For this review, take the finished solid that the model builds, in its own axes (mm). A direction names the side the tool comes from. Give positions to 0.01 mm unless a question says otherwise; leave off trailing zeros. Loops run counter-clockwise (first coordinate to the right, second up) from the corner with the lowest first, then second, coordinate; pieces in that order, holes last. Notation, with made-up numbers: (58.5, 65.5) - (89.5, 65.5) arc R26 ccw to (89.5, 79.5) - close; hole circle Ø3 at (46, -13). An arc over 180 degrees is marked (long way). Put each result on its own line as item: value.
from build123d import *

# Parameters (mm, degrees)
ESQUISSE1_R        = 1.75
BOSS_EXTRU_1_DEPTH = 10
BOSS_EXTRU_2_START = 25
ESQUISSE2_R        = 4
BOSS_EXTRU_2_DEPTH = 10
CHANFREIN1_SIZE    = 2
CONG_1_R           = 2


with BuildPart() as part:
    # Esquisse1 → Boss.-Extru.1 (new body)
    with BuildSketch(Plane.XY):
        with BuildLine():
            Line((-2.952917385, 110.865117237), (48.5, 73.209447125))
            Line((48.5, 73.209447125), (48.5, 41.690552875))
            Line((48.5, 41.690552875), (-2.952917385, 4.034882763))
            ThreePointArc((-2.952917385, 4.034882763), (-4.034882763, -2.952917385), (2.952917385, -4.034882763))
            Line((2.952917385, -4.034882763), (56.966203668, 35.494585987))
            Line((56.966203668, 35.494585987), (100.033796332, 35.494585987))
            Line((100.033796332, 35.494585987), (154.047082615, -4.034882763))
            ThreePointArc((154.047082615, -4.034882763), (161.034882763, -2.952917385), (159.952917385, 4.034882763))
            Line((159.952917385, 4.034882763), (108.5, 41.690552875))
            Line((108.5, 41.690552875), (108.5, 73.209447125))
            Line((108.5, 73.209447125), (159.952917385, 110.865117237))
            ThreePointArc((159.952917385, 110.865117237), (161.034882763, 117.852917385), (154.047082615, 118.934882763))
            Line((154.047082615, 118.934882763), (100.033796332, 79.405414013))
            Line((100.033796332, 79.405414013), (56.966203668, 79.405414013))
            Line((56.966203668, 79.405414013), (2.952917385, 118.934882763))
            ThreePointArc((2.952917385, 118.934882763), (-4.034882763, 117.852917385), (-2.952917385, 110.865117237))
        make_face()
        Circle(ESQUISSE1_R, mode=Mode.SUBTRACT)
        with Locations((0, 114.9)):
            Circle(ESQUISSE1_R, mode=Mode.SUBTRACT)
        with Locations((157, 0)):
            Circle(ESQUISSE1_R, mode=Mode.SUBTRACT)
        with Locations((157, 114.9)):
            Circle(ESQUISSE1_R, mode=Mode.SUBTRACT)
    extrude(amount=BOSS_EXTRU_1_DEPTH)

    # Esquisse2 → Boss.-Extru.2 (add)
    with BuildSketch(Plane(origin=(48.5, 158.810828025, 0), x_dir=(0, 0, 1), z_dir=(1, 0, 0)).offset(BOSS_EXTRU_2_START)):
        with BuildLine():
            Line((10, 111.360828025), (20, 111.360828025))
            ThreePointArc((20, 111.360828025), (30, 101.360828025), (20, 91.360828025))
            Line((20, 91.360828025), (10, 91.360828025))
            Line((10, 91.360828025), (10, 111.360828025))
        make_face()
        with Locations((20, 101.360828025)):
            Circle(ESQUISSE2_R, mode=Mode.SUBTRACT)
    extrude(amount=BOSS_EXTRU_2_DEPTH)

    # Chanfrein1
    chanfrein1_edges = [part.edges().sort_by_distance(p)[0] for p in [
        (134.226458693, 92.037282181, 10),
        (161.034882763, -2.952917385, 0),
        (127.040439473, 15.729851612, 0),
        (78.5, 35.494585987, 0),
        (161.034882763, 117.852917385, 10),
        (29.959560527, 15.729851612, 0),
        (-4.034882763, -2.952917385, 0),
        (22.773541307, 22.862717819, 0),
        (48.5, 57.45, 0),
        (22.773541307, 92.037282181, 0),
        (-4.034882763, 117.852917385, 0),
        (29.959560527, 99.170148388, 0),
        (78.5, 79.405414013, 0),
        (127.040439473, 99.170148388, 0),
        (161.034882763, 117.852917385, 0),
        (127.040439473, 99.170148388, 10),
        (134.226458693, 92.037282181, 0),
        (108.5, 57.45, 0),
        (134.226458693, 22.862717819, 0),
        (78.5, 79.405414013, 10),
        (29.959560527, 99.170148388, 10),
        (-4.034882763, 117.852917385, 10),
        (22.773541307, 92.037282181, 10),
        (48.5, 57.45, 10),
        (22.773541307, 22.862717819, 10),
        (-4.034882763, -2.952917385, 10),
        (134.226458693, 22.862717819, 10),
        (29.959560527, 15.729851612, 10),
        (78.5, 35.494585987, 10),
        (127.040439473, 15.729851612, 10),
        (161.034882763, -2.952917385, 10),
        (108.5, 57.45, 10),
    ]]
    chamfer(chanfrein1_edges, length=CHANFREIN1_SIZE)

    # Congé1
    cong_1_edges = [part.edges().sort_by_distance(p)[0] for p in [
        (83.5, 67.45, 15),
        (83.5, 57.45, 30),
        (83.5, 47.45, 15),
        (73.5, 67.45, 15),
        (73.5, 57.45, 30),
        (73.5, 47.45, 15),
    ]]
    fillet(cong_1_edges, radius=CONG_1_R)


solid = part.part
1) Insertion check: pin 1 Ø5.5 at (x, y) = (0, 114.9) entering from +Z; pin 2 Ø8 at (y, z) = (61, 15) entering from -X; pin 3 Ø6.5 at (y, z) = (57.45, 20) entering from +X; pin 4 Ø5 at (x, z) = (78, 16) entering from -Y. Each pin has a flat end and moves straight along its axis. Give the tip position at first contact, or say it passes through.
Geometry check:
pin 1: stops at z = 10
pin 2: stops at x = 73.5
pin 3: passes through
pin 4: stops at y = 47.45
2) Take a section at C-C on x = 157. State the section outline as (y, z) points, and give its area (3 significant figures).
Geometry check:
outline: (-5, 2) - (-3, 0) - (-1.75, 0) - (-1.75, 10) - (-3, 10) - (-5, 8) - close; (1.75, 0) - (3.72, 0) - (6.2, 2) - (6.2, 8) - (3.72, 10) - (1.75, 10) - close; (108.7, 2) - (111.18, 0) - (113.15, 0) - (113.15, 10) - (111.18, 10) - (108.7, 8) - close; (116.65, 0) - (117.9, 0) - (119.9, 2) - (119.9, 8) - (117.9, 10) - (116.65, 10) - close
area: 136 mm²
3) Take a section at D-D on x = 10. State the section outline as (y, z) points, and give its area (3 significant figures).
Geometry check:
outline: (1.12, 2) - (3.6, 0) - (11.04, 0) - (13.51, 2) - (13.51, 8) - (11.04, 10) - (3.6, 10) - (1.12, 8) - close; (101.39, 2) - (103.86, 0) - (111.3, 0) - (113.78, 2) - (113.78, 8) - (111.3, 10) - (103.86, 10) - (101.39, 8) - close
area: 228 mm²
4) Take a section at B-B on z = 5. State the section outline as (x, y) points.
Geometry check:
outline: (-2.95, 4.03) arc R5 ccw to (2.95, -4.03) - (56.97, 35.49) - (100.03, 35.49) - (154.05, -4.03) arc R5 ccw to (159.95, 4.03) - (108.5, 41.69) - (108.5, 73.21) - (159.95, 110.87) arc R5 ccw to (154.05, 118.93) - (100.03, 79.41) - (56.97, 79.41) - (2.95, 118.93) arc R5 ccw to (-2.95, 110.87) - (48.5, 73.21) - (48.5, 41.69) - close; hole circle Ø3.5 at (0, 0); hole circle Ø3.5 at (0, 114.9); hole circle Ø3.5 at (157, 0); hole circle Ø3.5 at (157, 114.9)
5) Wall thickness on line 1 (Y direction, x = 157, z = 8); line 2 (Z direction, x = 80.5, y = 57.45); line 3 (X direction, y = 25.5, z = 6): over which ranges is each line inside the solid? List them lowest first.
Geometry check:
line 1: y = -5 to -1.75, 1.75 to 6.2, 108.7 to 113.15, 116.65 to 119.9
line 2: z = 0 to 16, 24 to 30
line 3: x = 26.38 to 43.31, 113.69 to 130.62
6) For faces 4 (the face through (127.741, 98.461, 8.986)), 5 (the face through (79, 79.405, 5)), 6 (the face through (23.1, 23.1, 5)), list the 3-axis set-ups (+Z, -Z, +X, -X, +Y, -Y) from which the entire face can be reached by the end or side of a thin tool; tool diameter is ignored.
Geometry check:
face 4: +Z, +Y
face 5: +Z, -Z, +Y
face 6: +Z, -Z, -X
7) Draft analysis for pull direction X (two halves, no side actions). For faces 1 (the face through (84, 62, 10)), 2 (the face through (133.601, 22.099, 1.014)), 3 (the face through (127.741, 98.461, 1.014)), state which applies: pulls with the +X half, pulls with the -X half, needs draft (parallel to the pull), parting line crosses it, or undercut.
Geometry check:
face 1: needs draft
face 2: pulls with the +X half
face 3: undercut
8) Take a section at A-A on y = 57.45. State the section outline as (x, z) points.
Geometry check:
outline: (48.5, 2) - (50.5, 0) - (106.5, 0) - (108.5, 2) - (108.5, 8) - (106.5, 10) - (83.5, 10) - (83.5, 16) - (73.5, 16) - (73.5, 10) - (50.5, 10) - (48.5, 8) - close; (73.5, 24) - (83.5, 24) - (83.5, 28) arc R2 ccw to (81.5, 30) - (75.5, 30) arc R2 ccw to (73.5, 28) - close
